CAD build for the part. Positions are in the model's coordinates, mm. Give positions to 0.01 mm unless a question says otherwise; leave off trailing zeros. Order: outer loops, then holes, each group sorted by start corner. A loop starts at its lowest first (then second) coordinate and runs counter-clockwise, first axis right, second up.
Autodesk Inventor part; units mm, degrees
ref_plane "YZ Plane" through (0, 0, 0) normal (1, 0, 0) x (0, 1, 0)
ref_plane "XZ Plane" through (0, 0, 0) normal (0, 1, 0) x (-1, 0, 0)
ref_plane "XY Plane" through (0, 0, 0) normal (0, 0, 1) x (1, 0, 0)
sketch "スケッチ1" plane through (0, 0, 0) normal (0, 1, 0) x (-1, 0, 0)
  line L0 (-68, -11.5) -> (68, -11.5)
  line L1 (68, -11.5) -> (68, 11.5)
  line L2 (68, 11.5) -> (-68, 11.5)
  line L3 (-68, 11.5) -> (-68, -11.5)
  line L4 (-68, -11.5) -> (68, 11.5) construction
  line L5 (68, -11.5) -> (-68, 11.5) construction
  point P0 (0, 0)
  dimension "d0" = 136
  dimension "d1" = 23
extrude "押し出し1" add sketch "スケッチ1" along normal blind 5.5
chamfer "面取り1" distance 20 distance2 10 1 edges at (68, 2.75, 11.5) measured on face at (-22.6667, 3.6667, 11.5)
properties part number "stopper" material "木材 (カエデ材)"
1. Saw through at C-C on z = 7. Give the cut face in (x, y), plus the area to 4 significant figures.
2. Saw through at A-A on x = 53. Give the cut face in (y, z).
3. Saw through at B-B on y = 3.5. Give the cut face in (x, z).
4. Wall check: line 1 (X direction, y = 3.05, z = 4.25); line 2 (X direction, y = 1.3, z = 3); line 3 (Z direction, x = 62, y = 1.3). Give the ranges that are in metal, low to high.
Reported:
1. outline: (-68, 0) - (57, 0) - (57, 5.5) - (-68, 5.5) - close
1. area: 687.5 mm2
2. outline: (0, -11.5) - (5.5, -11.5) - (5.5, 9) - (0, 9) - close
3. outline: (-68, -11.5) - (68, -11.5) - (68, 1.5) - (48, 11.5) - (-68, 11.5) - close
4. line 1: x = -68 to 62.5
4. line 2: x = -68 to 65
4. line 3: z = -11.5 to 4.5
